For this review, take the finished solid that the model builds, in its own axes (mm). A direction names the side the tool comes from. Coordinates: 2 decimals unless noted, no trailing zeros. Loops run counter-clockwise (first coordinate to the right, second up) from the corner with the lowest first, then second, coordinate; pieces in that order, holes last.
1. To check wall thickness, follow probe 1 along Y at (x, z) = (-11.3, 6.5); probe 2 along Z at (x, y) = (0.5, 44.5); probe 3 along X at (y, z) = (24, 5.5). State the ranges of each line that lie inside material, in increasing order.
2. Machinability: for faces 1 (the face through (8.13, 25.4, 6.56)), 2 (the face through (-16.43, 20.4, 11.4)), 3 (the face through (9.54, 53.7, 9.5)), which of the approach directions +Z, -Z, +X, -X, +Y, -Y give a long, thin tool a straight path to every point of the face, cutting with its end or side? Answer none if there is none.
3. Take a section at C-C, the plane y = 50. State the section outline as (x, z) points.
4. Take a section at A-A, the plane y = 22. State the section outline as (x, z) points, then the cut area to 3 significant figures.
5. Clearance check with flat-ended pins moving along their axes: P1, Ø4, axis at y = 60, z = 6.5, coming from the -X side; P2, Ø0.5, axis at x = 1, z = 12.5, coming from the -Y side; P3, Ø8, axis at y = 49.5, z = 8, coming from the +X side. State where each tip first meets the part, or that it passes through.
6. Mouldability with a two-part tool opening along Z and no side actions: class faces 4 (the face through (0, 30, 7)), 5 (the face through (0, 26, 6)), 6 (the face through (-0.2, 27.5, 1)), 7 (the face through (-0.2, 27.5, 12)) as pulls with the +Z half, pulls with the -Z half, needs draft (parallel to the pull), parting line crosses it, or undercut.
```python
from build123d import *

# Parameters (mm, degrees)
CYLINDER013_R     = 1.2
CYLINDER013_DEPTH = 30
CYLINDER010_R     = 2
CYLINDER010_DEPTH = 50
BOX003_W          = 17.4
BOX003_H          = 26
BOX003_DEPTH      = 13
FILLET012_R       = 2
CYLINDER011_R     = 10
CYLINDER011_DEPTH = 40
CHAMFER008_SIZE   = 9
CYLINDER012_R     = 13
CYLINDER012_DEPTH = 40
CHAMFER009_SIZE   = 4
FILLET016_R       = 6
FILLET017_R       = 5
BOX004_W          = 34
BOX004_H          = 30
BOX004_DEPTH      = 11
FILLET013_R       = 5
CHAMFER010_SIZE   = 10
FILLET018_R       = 20
FILLET019_R       = 2
FILLET020_R       = 2
FILLET021_R       = 1


with BuildPart() as cylinder013:
    # Cylinder013 → Cylinder013 (new body)
    with BuildSketch(Plane(origin=(-15, 60, 6.5), x_dir=(0, 0, -1), z_dir=(1, 0, 0))):
        Circle(CYLINDER013_R)
    extrude(amount=CYLINDER013_DEPTH)


with BuildPart() as cylinder010:
    # Cylinder010 → Cylinder010 (new body)
    with BuildSketch(Plane(origin=(-25, 18, 6.5), x_dir=(0, 0, -1), z_dir=(1, 0, 0))):
        Circle(CYLINDER010_R)
    extrude(amount=CYLINDER010_DEPTH)


with BuildPart() as fillet012:
    # Box003 → Box003 (new body)
    with BuildSketch(Plane(origin=(-8.7, 0, 0), x_dir=(1, 0, 0), z_dir=(0, 0, 1))):
        with Locations((8.7, 13)):
            Rectangle(BOX003_W, BOX003_H)
    extrude(amount=BOX003_DEPTH)

    # Fillet012
    fillet012_edges = [fillet012.edges().sort_by_distance(p)[0] for p in [
        (-8.7, 26, 6.5),
        (8.7, 26, 6.5),
    ]]
    fillet(fillet012_edges, radius=FILLET012_R)


with BuildPart() as fusion005:
    # Cylinder011 → Cylinder011 (new body)
    with BuildSketch(Plane(origin=(0, 70, 6.5), x_dir=(1, 0, 0), z_dir=(0, -1, 0))):
        Circle(CYLINDER011_R)
    extrude(amount=CYLINDER011_DEPTH)

    # Chamfer008
    chamfer008_edges = [fusion005.edges().sort_by_distance(p)[0] for p in [
        (-10, 30, 6.5),
    ]]
    chamfer(chamfer008_edges, length=CHAMFER008_SIZE)

    # Fusion005: union Cylinder013, Cylinder010, Fillet012
    add(cylinder013.part)
    add(cylinder010.part)
    add(fillet012.part)


with BuildPart() as fillet017:
    # Cylinder012 → Cylinder012 (new body)
    with BuildSketch(Plane(origin=(0, 68, 6.5), x_dir=(1, 0, 0), z_dir=(0, -1, 0))):
        Circle(CYLINDER012_R)
    extrude(amount=CYLINDER012_DEPTH)

    # Chamfer009
    chamfer009_edges = [fillet017.edges().sort_by_distance(p)[0] for p in [
        (-13, 28, 6.5),
    ]]
    chamfer(chamfer009_edges, length=CHAMFER009_SIZE)

    # Fillet016
    fillet016_edges = [fillet017.edges().sort_by_distance(p)[0] for p in [
        (-9, 28, 6.5),
    ]]
    fillet(fillet016_edges, radius=FILLET016_R)

    # Fillet017
    fillet017_edges = [fillet017.edges().sort_by_distance(p)[0] for p in [
        (-13, 32, 6.5),
    ]]
    fillet(fillet017_edges, radius=FILLET017_R)


with BuildPart() as obj1:
    # Box004 → Box004 (new body)
    with BuildSketch(Plane(origin=(-17, 12, 1), x_dir=(1, 0, 0), z_dir=(0, 0, 1))):
        with Locations((17, 15)):
            Rectangle(BOX004_W, BOX004_H)
    extrude(amount=BOX004_DEPTH)

    # Fillet013
    fillet013_edges = [obj1.edges().sort_by_distance(p)[0] for p in [
        (0, 12, 1),
        (0, 12, 12),
    ]]
    fillet(fillet013_edges, radius=FILLET013_R)

    # Chamfer010
    chamfer010_edges = [obj1.edges().sort_by_distance(p)[0] for p in [
        (-17, 42, 6.5),
        (17, 42, 6.5),
    ]]
    chamfer(chamfer010_edges, length=CHAMFER010_SIZE)

    # Fillet018
    fillet018_edges = [obj1.edges().sort_by_distance(p)[0] for p in [
        (-17, 32, 6.5),
        (17, 32, 6.5),
    ]]
    fillet(fillet018_edges, radius=FILLET018_R)

    # Fillet019
    fillet019_edges = [obj1.edges().sort_by_distance(p)[0] for p in [
        (15.477591, 31.369397, 12),
    ]]
    fillet(fillet019_edges, radius=FILLET019_R)

    # Fillet020
    fillet020_edges = [obj1.edges().sort_by_distance(p)[0] for p in [
        (-15.477591, 31.369397, 12),
    ]]
    fillet(fillet020_edges, radius=FILLET020_R)

    # Fusion006: union Fillet017
    add(fillet017.part)

    # Cut005: cut Fusion005
    add(fusion005.part, mode=Mode.SUBTRACT)

    # Fillet021
    fillet021_edges = [obj1.edges().sort_by_distance(p)[0] for p in [
        (0, 26, 12),
    ]]
    fillet(fillet021_edges, radius=FILLET021_R)


solid = obj1.part
```
Results list:
1. probe 1: y = 12 to 16, 20 to 58.8, 61.2 to 68
1. probe 2: z = -6.49 to -3.49, 16.49 to 19.49
1. probe 3: x = -17 to -8.7, 8.7 to 17
2. face 1: +Z, -Z, -Y
2. face 2: +Z, -X, +Y, -Y
2. face 3: +Y
3. outline: circle Ø26 at (0, 6.5); hole circle Ø20 at (0, 6.5)
4. outline: (-17, 3) arc R2 ccw to (-15, 1) - (-9.7, 1) arc R1 ccw to (-8.7, 2) - (-8.7, 11) arc R1 ccw to (-9.7, 12) - (-15, 12) arc R2 ccw to (-17, 10) - close; (8.7, 2) arc R1 ccw to (9.7, 1) - (15, 1) arc R2 ccw to (17, 3) - (17, 10) arc R2 ccw to (15, 12) - (9.7, 12) arc R1 ccw to (8.7, 11) - close
4. area: 178 mm2
5. P1: stops at x = -13
5. P2: stops at y = 28
5. P3: stops at x = 13
6. face 4: undercut
6. face 5: needs draft
6. face 6: pulls with the -Z half
6. face 7: pulls with the +Z half
